from build123d import *

# Parameters (mm, degrees)
BOSS_EXTRUDE2_DEPTH     = 105
BOSS_EXTRUDE3_DEPTH     = 54
SKETCH3_4_W             = 80
SKETCH3_4_H             = 45
BOSS_EXTRUDE4_DEPTH     = 62
CUT_EXTRUDE1_DEPTH      = 18.5
CUT_EXTRUDE1_DEPTH_BACK = 98.5
FILLET1_R               = 20
SKETCH7_R               = 15
CUT_EXTRUDE2_DEPTH      = 160


with BuildPart() as part:
    # Sketch3 → Boss-Extrude2 (new body, symmetric)
    with BuildSketch(Plane.XY):
        Polygon((30, -161.018016556), (-30, -161.018016556), (-57.5, -161.018016556), (-57.5, -191.018016556), (57.5, -191.018016556), (57.5, -161.018016556), align=None)
    extrude(amount=BOSS_EXTRUDE2_DEPTH, both=True)

    # Sketch3<3> → Boss-Extrude3 (add, symmetric)
    with BuildSketch(Plane.XY):
        with BuildLine():
            Line((-40, 107.819293264), (-40, -107.819293264))
            ThreePointArc((-40, -107.819293264), (-35.036523196, -109.532835453), (-30, -111.018016556))
            Line((-30, -111.018016556), (-30, -161.018016556))
            Line((-30, -161.018016556), (30, -161.018016556))
            Line((30, -161.018016556), (30, -111.018016556))
            ThreePointArc((30, -111.018016556), (35.036523196, -109.532835453), (40, -107.819293264))
            Line((40, -107.819293264), (40, 107.819293264))
            ThreePointArc((40, 107.819293264), (0, 115), (-40, 107.819293264))
        make_face()
    extrude(amount=BOSS_EXTRUDE3_DEPTH, both=True)

    # Sketch3<4> → Boss-Extrude4 (add)
    with BuildSketch(Plane.XY):
        Rectangle(SKETCH3_4_W, SKETCH3_4_H)
    extrude(amount=BOSS_EXTRUDE4_DEPTH)

    # Sketch5 → Cut-Extrude1 (cut, two sides)
    with BuildSketch(Plane(origin=(40, 0, 0), x_dir=(0, 0, -1), z_dir=(1, 0, 0))) as cut_extrude1_sk:
        with BuildLine():
            Line((54, 43.981983444), (-6, 43.981983444))
            ThreePointArc((-6, 43.981983444), (-46, 3.981983444), (-6, -36.018016556))
            Line((-6, -36.018016556), (54, -36.018016556))
            Line((54, -36.018016556), (54, 43.981983444))
        make_face()
    extrude(amount=CUT_EXTRUDE1_DEPTH, mode=Mode.SUBTRACT)
    extrude(cut_extrude1_sk.sketch, amount=-CUT_EXTRUDE1_DEPTH_BACK, mode=Mode.SUBTRACT)

    # Fillet1
    fillet1_edges = [part.edges().sort_by_distance(p)[0] for p in [
        (0, -161.018016556, -54),
        (-30, -161.018016556, 0),
        (30, -161.018016556, 0),
        (0, -161.018016556, 54),
    ]]
    fillet(fillet1_edges, radius=FILLET1_R)

    # Sketch7 → Cut-Extrude2 (cut, through all)
    with BuildSketch(Plane.XY.offset(54)):
        with Locations((0, -71.018016556)):
            Circle(SKETCH7_R)
        with Locations((0, 78.981983444)):
            Circle(SKETCH7_R)
    extrude(amount=-CUT_EXTRUDE2_DEPTH, mode=Mode.SUBTRACT)


solid = part.part
Check sheet for the modelled part. Datum: model origin and axes. Units: mm. A direction names the side the tool comes from. Round coordinates to 2 decimals unless told otherwise and drop trailing zeros. Loops run counter-clockwise (first coordinate to the right, second up) from the corner with the lowest first, then second, coordinate; pieces in that order, holes last.
1. Scan lines: probe 1 along Y at (x, z) = (0, -8); probe 2 along Y at (x, z) = (-33.5, -40); probe 3 along Y at (x, z) = (10.5, 0.5). Record each from-to range of solid material in increasing order.
2. Sectioned sample at D-D on z = 67.5. Record the boundary of the cut face in (x, y).
3. Set-up check for faces 1 (the flat face through (-1, -22.5, 58)), 2 (the flat face through (-50.3, -161.018, 1.5)), 3 (the cylindrical face through (34.966, -109.555, 0.756)): record each of +Z, -Z, +X, -X, +Y, -Y from which the full face is reachable in a straight line by a thin tool's end or side.
4. Gauge pin test, flat ends, axial feed: pin 1 Ø2 at (x, y) = (-15.5, -100.5) entering from +Z; pin 2 Ø24 at (x, y) = (16, -88) entering from -Z; pin 3 Ø24 at (y, z) = (-130.5, -9) entering from -X (3 decimals); pin 4 Ø24 at (x, y) = (1.5, 78) entering from +Z. Record the tip position at first contact, or that the pin passes through.
5. Sectioned sample at A-A on z = 25.5. Record the boundary of the cut face in (x, y), and give its area (3 significant figures).
6. Mould release check, pull along Y, two halves, no side actions. Record for faces 4 (the flat face through (-1, 22.5, 58)), 5 (the flat face through (40, 22, 43)), 6 (the flat face through (1, -36.018, -24)): released by +Y, released by -Y, zero draft, split by the parting line, or undercut.
7. Sectioned sample at B-B on x = 0. Record the boundary of the cut face in (y, z), and give its area (3 significant figures).
8. Sectioned sample at C-C on y = -64.5. Record the boundary of the cut face in (x, z), and give its area (3 significant figures).
Recorded:
1. probe 1: y = -191.02 to -86.02, -56.02 to -36.02, 43.98 to 63.98, 93.98 to 115
1. probe 2: y = -191.02 to -152.32, -110.01 to -36.02, 43.98 to 110.01
1. probe 3: y = -191.02 to -81.73, -60.31 to -36.02, 43.98 to 68.27, 89.69 to 114.52
2. outline: (-57.5, -191.02) - (57.5, -191.02) - (57.5, -161.02) - (50, -161.02) arc R20 cw to (43.5, -159.93) - (-43.5, -159.93) arc R20 cw to (-50, -161.02) - (-57.5, -161.02) - close
3. face 1: +Z, +X, -X
3. face 2: +Y
3. face 3: +Z, -Z, +X
4. pin 1: stops at z = 54
4. pin 2: stops at z = -54
4. pin 3: stops at x = -30.055
4. pin 4: passes through
5. outline: (-57.5, -191.02) - (57.5, -191.02) - (57.5, -161.02) - (50, -161.02) arc R20 cw to (30, -141.02) - (30, -111.02) arc R115 ccw to (40, -107.82) - (40, -30.94) - (-40, -30.94) - (-40, -107.82) arc R115 ccw to (-30, -111.02) - (-30, -141.02) arc R20 cw to (-50, -161.02) - (-57.5, -161.02) - close; (-40, 38.91) - (40, 38.91) - (40, 107.82) arc R115 ccw to (-40, 107.82) - close; hole circle Ø30 at (0, -71.02); hole circle Ø30 at (0, 78.98)
5. area: 17,500 mm2
6. face 4: released by +Y
6. face 5: zero draft
6. face 6: undercut
7. outline: (-191.02, -105) - (-161.02, -105) - (-161.02, -74) arc R20 cw to (-141.02, -54) - (-86.02, -54) - (-86.02, 54) - (-141.02, 54) arc R20 cw to (-161.02, 74) - (-161.02, 105) - (-191.02, 105) - close; (-56.02, -54) - (-36.02, -54) - (-36.02, 6) arc R40 cw to (43.98, 6) - (43.98, -54) - (63.98, -54) - (63.98, 54) - (22.5, 54) - (22.5, 62) - (-22.5, 62) - (-22.5, 54) - (-56.02, 54) - close; (93.98, -54) - (115, -54) - (115, 54) - (93.98, 54) - close
7. area: 22,800 mm2
8. outline: (-40, -54) - (-13.51, -54) - (-13.51, 54) - (-40, 54) - close; (13.51, -54) - (40, -54) - (40, 54) - (13.51, 54) - close
8. area: 5,720 mm2
